```python
from build123d import *

# Parameters (mm, degrees)
EXTRUDE1_DEPTH = 17
FILLET1_R      = 10
SKETCH2_R      = 2.5
EXTRUDE2_DEPTH = 17
SKETCH3_R      = 2.5
EXTRUDE3_DEPTH = 17


with BuildPart() as part:
    # Sketch1 → Extrude1 (new body)
    with BuildSketch(Plane.XY):
        Polygon((-145.737121951, 14.824159554), (4.262878049, 14.824159554), (19.262878049, 38.324159554), (94.262878049, 38.324159554), (94.262878049, 31.324159554), (24.769095529, 31.324159554), (9.769095529, 7.824159554), (-145.737121951, 7.824159554), align=None)
    extrude(amount=EXTRUDE1_DEPTH)

    # Fillet1
    fillet1_edges = [part.edges().sort_by_distance(p)[0] for p in [
        (4.262878049, 14.824159554, 8.5),
        (19.262878049, 38.324159554, 8.5),
        (24.769095529, 31.324159554, 8.5),
        (9.769095529, 7.824159554, 8.5),
    ]]
    fillet(fillet1_edges, radius=FILLET1_R)

    # Sketch2 → Extrude2 (cut)
    with BuildSketch(Plane(origin=(0, 38.324159554, 0), x_dir=(1, 0, 0), z_dir=(0, 1, 0))):
        with Locations((79.262878049, -8.5)):
            Circle(SKETCH2_R)
        with Locations((64.262878049, -8.5)):
            Circle(SKETCH2_R)
    extrude(amount=-EXTRUDE2_DEPTH, mode=Mode.SUBTRACT)

    # Sketch3 → Extrude3 (cut)
    with BuildSketch(Plane.XZ.offset(-7.824159554)):
        with Locations((-140.737121951, 8.5)):
            Circle(SKETCH3_R)
    extrude(amount=-EXTRUDE3_DEPTH, mode=Mode.SUBTRACT)


solid = part.part
```
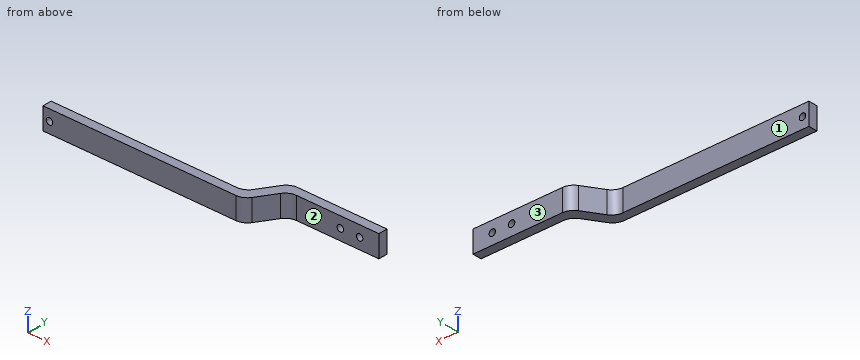
CAD build for the part. Positions are in the model's coordinates, mm. Face numbers are marked on the shaded views. A direction names the side the tool comes from. Coordinates: 2 decimals unless noted, no trailing zeros. Order: outer loops, then holes, each group sorted by start corner. A loop starts at its lowest first (then second) coordinate and runs counter-clockwise, first axis right, second up. Notation, with made-up numbers: M -14.5,18 L 0.5,18 A22 cw 0.5,51 Z; hole C 3.5,77.25 d8. An arc over 180 degrees is marked long. Answer as CSV lines item,"result".
1) Cut at B-B (x = -86.5). List the corners of the cut face in (y, z), then the cut area to 3 significant figures.
Verdict:
outline,"M 7.82,0 L 14.82,0 L 14.82,17 L 7.82,17 Z"
area,"119 mm2"
2) 3-axis set-ups, long thin cutter, end or side, ignore diameter. For the marked faces 1, 2 and 3: which of +Z, -Z, +X, -X, +Y, -Y reach the whole face in a straight line?
Verdict:
face 1,"+Z, -Z, -X, +Y"
face 2,"+Z, -Z, +X, -Y"
face 3,"+Z, -Z, +X, -X, +Y"
3) Flat gauge pins, fed straight in: P1, Ø2, axis at x = -51, y = 17, coming from the -Z side; P2, Ø5, axis at y = 16.5, z = 11.5, coming from the +X side; P3, Ø10, axis at x = -86, z = 3.5, coming from the +Y side; P4, Ø8.5, axis at x = 70.5, z = 9, coming from the -Y side. Where does each tip first touch, or does it go through?
Verdict:
P1,"through"
P2,"x = 16.9"
P3,"y = 14.82"
P4,"y = 31.32"
4) Cut at A-A (z = 8.5). List the corners of the cut face in (x, y), then the cut area to 3 significant figures.
Verdict:
outline,"M -145.74,7.82 L -143.24,7.82 L -143.24,14.82 L -145.74,14.82 Z; M -138.24,7.82 L 4.29,7.82 A10 ccw 12.72,12.44 L 21.82,26.7 A10 cw 30.25,31.32 L 61.76,31.32 L 61.76,38.32 L 24.74,38.32 A10 ccw 16.31,33.7 L 7.21,19.44 A10 cw -1.22,14.82 L -138.24,14.82 Z; M 66.76,31.32 L 76.76,31.32 L 76.76,38.32 L 66.76,38.32 Z; M 81.76,31.32 L 94.26,31.32 L 94.26,38.32 L 81.76,38.32 Z"
area,"1,700 mm2"
5) Drill centre lines: L1, parallel to X at y = 33.25, z = 8.5; L2, parallel to X at y = 35, z = 8.5; L3, parallel to Y at x = -73.5, z = 15.25. Where is each one in solid material? Low to high. Write a range as from..to.
Verdict:
L1,"16.02..61.76, 66.76..76.76, 81.76..94.26"
L2,"17.3..61.76, 66.76..76.76, 81.76..94.26"
L3,"7.82..14.82"
